Could you check a few things on this model? Use its own coordinates, in mm. A direction names the side the tool comes from. Give positions to 0.01 mm unless a question says otherwise; leave off trailing zeros. Loops run counter-clockwise (first coordinate to the right, second up) from the corner with the lowest first, then second, coordinate; pieces in that order, holes last. Notation, with made-up numbers: (38.5, 39.25) -> (77.5, 39.25) arc R9 ccw to (77.5, 54.25) -> close; hole circle Ø4 at (39, -16.75). An arc over 180 degrees is marked (long way). Put each result on its own line as item: value.
```python
from build123d import *

# Parameters (mm, degrees)
SKETCH_1_W               = 90
SKETCH_1_H               = 65
EXTRUDE_1_DEPTH          = 2
SKETCH_2_W               = 52
SKETCH_2_H               = 13
CUT_EXTRUDE_1_DEPTH      = 56.54502678
CUT_EXTRUDE_2_DEPTH      = 56.54502678
MIRROR_3_COPY_1_DEPTH    = 56.54502678
FILLET_1_R               = 7
SKETCH_4_W               = 41
SKETCH_4_H               = 2
EXTRUDE_2_DEPTH          = 73
SKETCH_5_W               = 15
SKETCH_5_H               = 59.991373208
CUT_EXTRUDE_3_DEPTH      = 0.5
FILLET_2_R               = 0.5
FILLET_3_R               = 0.5
CHAMFER_4_SIZE           = 12
CHAMFER_4_SIZE2          = 25.734083046
CHAMFER_5_SIZE           = 12
CHAMFER_5_SIZE2          = 25.734083046
CHAMFER_6_SIZE           = 12
CHAMFER_6_SIZE2          = 25.734083046
CHAMFER_7_SIZE           = 12
CHAMFER_7_SIZE2          = 25.734083046
FILLET_4_R               = 10
EXTRUDE_3_DEPTH          = 6
EXTRUDE_START            = -41
SKETCH_7_R               = 4
EXTRUDE_4_DEPTH          = 42
SKETCH_8_R               = 2.75
CUT_EXTRUDE_4_DEPTH      = 92.707415265
MIRROR_9_COPY_1_SKETCH_R = 2.75
MIRROR_9_COPY_1_DEPTH    = 92.707415265
EXTRUDE_7_DEPTH          = 13
EXTRUDE_7_DEPTH_BACK     = 13
SKETCH_10_R              = 37.5
FILLET_5_R               = 2
SKETCH_11_R              = 25
SKETCH_11_R_2            = 22
CUT_EXTRUDE_5_DEPTH      = 3
FILLET_6_R               = 2
FILLET_7_R               = 2
CHAMFER_8_SIZE2          = 5.196152423
CHAMFER_8_SIZE           = 3
CHAMFER_9_SIZE2          = 3
CHAMFER_9_SIZE           = 5.196152423


with BuildPart() as part:
    # 草图1 → 凸台-拉伸1 (new body)
    with BuildSketch(Plane.XY):
        Rectangle(SKETCH_1_W, SKETCH_1_H)
    extrude(amount=EXTRUDE_1_DEPTH)

    # 草图2 → 切除-拉伸1 (cut, through all)
    with BuildSketch(Plane.XY.offset(2)):
        with Locations((0, 26)):
            Rectangle(SKETCH_2_W, SKETCH_2_H)
    cut_extrude_1 = extrude(amount=-CUT_EXTRUDE_1_DEPTH, mode=Mode.SUBTRACT)

    # 镜向1: 切除-拉伸1 across plane
    add(cut_extrude_1.mirror(Plane.ZX), mode=Mode.SUBTRACT)

    # 草图3 → 切除-拉伸2 (cut, through all)
    with BuildSketch(Plane.XY.offset(2)):
        with BuildLine():
            Line((-36.562223186, 30.159744382), (-34.562223186, 30.159744382))
            ThreePointArc((-34.562223186, 30.159744382), (-30.562223186, 26.159744382), (-34.562223186, 22.159744382))
            Line((-34.562223186, 22.159744382), (-36.562223186, 22.159744382))
            ThreePointArc((-36.562223186, 22.159744382), (-40.562223186, 26.159744382), (-36.562223186, 30.159744382))
        make_face()
    cut_extrude_2 = extrude(amount=-CUT_EXTRUDE_2_DEPTH, mode=Mode.SUBTRACT)

    # 镜向2: 切除-拉伸2 across plane
    add(cut_extrude_2.mirror(Plane(origin=(0, 0, 0), x_dir=(0, 0, 1), z_dir=(1, 0, 0))), mode=Mode.SUBTRACT)

    # 镜向3: 切除-拉伸2 across plane
    add(cut_extrude_2.mirror(Plane.ZX), mode=Mode.SUBTRACT)

    # 镜向3 copy 1 sketch → 镜向3 copy 1 (cut, through all)
    with BuildSketch(Plane(origin=(0, 0, 2), x_dir=(-1, 0, 0), z_dir=(0, 0, 1))):
        with BuildLine():
            Line((-36.562223186, 30.159744382), (-34.562223186, 30.159744382))
            ThreePointArc((-34.562223186, 30.159744382), (-30.562223186, 26.159744382), (-34.562223186, 22.159744382))
            Line((-34.562223186, 22.159744382), (-36.562223186, 22.159744382))
            ThreePointArc((-36.562223186, 22.159744382), (-40.562223186, 26.159744382), (-36.562223186, 30.159744382))
        make_face()
    extrude(amount=-MIRROR_3_COPY_1_DEPTH, mode=Mode.SUBTRACT)

    # 圆角1
    fillet_1_edges = [part.edges().sort_by_distance(p)[0] for p in [
        (-26, 32.5, 1),
        (26, 32.5, 1),
        (-26, -32.5, 1),
        (26, -32.5, 1),
        (45, -32.5, 1),
        (-45, -32.5, 1),
        (-45, 32.5, 1),
        (45, 32.5, 1),
    ]]
    fillet(fillet_1_edges, radius=FILLET_1_R)

    # 草图4 → 凸台-拉伸2 (add)
    with BuildSketch(Plane(origin=(0, 0, 0), x_dir=(-1, 0, 0), z_dir=(0, 0, -1))):
        with Locations((0, 18.5)):
            Rectangle(SKETCH_4_W, SKETCH_4_H)
    extrude_2 = extrude(amount=EXTRUDE_2_DEPTH)

    # 镜向4: 凸台-拉伸2 across plane
    add(extrude_2.mirror(Plane.ZX))

    # 草图5 → 切除-拉伸3 (cut)
    with BuildSketch(Plane(origin=(0, 19.5, 0), x_dir=(1, 0, 0), z_dir=(0, 1, 0))):
        with Locations((0, 43.004313396)):
            Rectangle(SKETCH_5_W, SKETCH_5_H)
    cut_extrude_3 = extrude(amount=-CUT_EXTRUDE_3_DEPTH, mode=Mode.SUBTRACT)

    # 圆角2
    fillet_2_edges = [part.edges().sort_by_distance(p)[0] for p in [
        (0, 19.5, -13.008626792),
        (7.5, 19.5, -43.004313396),
        (-7.5, 19.5, -43.004313396),
    ]]
    fillet(fillet_2_edges, radius=FILLET_2_R - 0.0001)  # a hair under: the kernel refuses the full size

    # 镜向6: 切除-拉伸3 across plane
    add(cut_extrude_3.mirror(Plane.ZX), mode=Mode.SUBTRACT)

    # 圆角3
    fillet_3_edges = [part.edges().sort_by_distance(p)[0] for p in [
        (7.5, -19.5, -43.004313396),
        (-7.5, -19.5, -43.004313396),
        (0, -19.5, -13.008626792),
    ]]
    fillet(fillet_3_edges, radius=FILLET_3_R - 0.0001)  # a hair under: the kernel refuses the full size

    # 倒角4
    chamfer_4_edges = [part.edges().sort_by_distance(p)[0] for p in [
        (-20.5, -18.5, -73),
    ]]
    chamfer_4_side = [part.faces().sort_by_distance(p)[0] for p in [
        (0, -18.423106996, -73),
    ]]
    chamfer(chamfer_4_edges, length=CHAMFER_4_SIZE, length2=CHAMFER_4_SIZE2, reference=chamfer_4_side[0])

    # 倒角5
    chamfer_5_edges = [part.edges().sort_by_distance(p)[0] for p in [
        (20.5, -18.5, -73),
    ]]
    chamfer_5_side = [part.faces().sort_by_distance(p)[0] for p in [
        (6.905756389, -18.386486006, -73),
    ]]
    chamfer(chamfer_5_edges, length=CHAMFER_5_SIZE, length2=CHAMFER_5_SIZE2, reference=chamfer_5_side[0])

    # 倒角6
    chamfer_6_edges = [part.edges().sort_by_distance(p)[0] for p in [
        (20.5, 18.5, -73),
    ]]
    chamfer_6_side = [part.faces().sort_by_distance(p)[0] for p in [
        (0, 18.423106996, -73),
    ]]
    chamfer(chamfer_6_edges, length=CHAMFER_6_SIZE, length2=CHAMFER_6_SIZE2, reference=chamfer_6_side[0])

    # 倒角7
    chamfer_7_edges = [part.edges().sort_by_distance(p)[0] for p in [
        (-20.5, 18.5, -73),
    ]]
    chamfer_7_side = [part.faces().sort_by_distance(p)[0] for p in [
        (-6.905756389, 18.386486006, -73),
    ]]
    chamfer(chamfer_7_edges, length=CHAMFER_7_SIZE, length2=CHAMFER_7_SIZE2, reference=chamfer_7_side[0])

    # 圆角4
    fillet_4_edges = [part.edges().sort_by_distance(p)[0] for p in [
        (-8.5, 18.5, -73),
        (8.5, 18.5, -73),
        (8.5, -18.5, -73),
        (-8.5, -18.5, -73),
    ]]
    fillet(fillet_4_edges, radius=FILLET_4_R)

    # 草图6 → 凸台-拉伸3 (add)
    with BuildSketch(Plane(origin=(0, 19, 0), x_dir=(1, 0, 0), z_dir=(0, 1, 0))):
        Polygon((-4.39108988, 69.342635878), (-7.986809677, 62.196252237), (-3.595719796, 55.509075728), (4.39108988, 55.96828286), (7.986809677, 63.114666501), (3.595719796, 69.801843011), align=None)
    extrude_3 = extrude(amount=EXTRUDE_3_DEPTH)

    # 草图7 → 凸台-拉伸4 (add)
    with BuildSketch(Plane(origin=(0, 25, 0), x_dir=(1, 0, 0), z_dir=(0, 1, 0)).offset(EXTRUDE_START)):
        with Locations(Location((0, 62.655459369, 0), (0, 0, 270))):
            Circle(SKETCH_7_R)
    extrude_4 = extrude(amount=EXTRUDE_4_DEPTH)

    # 镜向7: 凸台-拉伸3, 凸台-拉伸4 across plane
    add(extrude_3.mirror(Plane.ZX))
    add(extrude_4.mirror(Plane.ZX))

    # 草图8 → 切除-拉伸4 (cut, through all)
    with BuildSketch(Plane(origin=(0, 0, 0), x_dir=(-1, 0, 0), z_dir=(0, 0, -1))):
        with Locations((-23.25, 19.5)):
            Circle(SKETCH_8_R)
    cut_extrude_4 = extrude(amount=-CUT_EXTRUDE_4_DEPTH, mode=Mode.SUBTRACT)

    # 镜向8: 切除-拉伸4 across plane
    add(cut_extrude_4.mirror(Plane.ZX), mode=Mode.SUBTRACT)

    # 镜向9: 切除-拉伸4 across plane
    add(cut_extrude_4.mirror(Plane(origin=(0, 0, 0), x_dir=(0, 0, 1), z_dir=(1, 0, 0))), mode=Mode.SUBTRACT)

    # 镜向9 copy 1 sketch → 镜向9 copy 1 (cut, through all)
    with BuildSketch(Plane(origin=(0, 0, 0), x_dir=(1, 0, 0), z_dir=(0, 0, -1))):
        with Locations((-23.25, 19.5)):
            Circle(MIRROR_9_COPY_1_SKETCH_R)
    extrude(amount=-MIRROR_9_COPY_1_DEPTH, mode=Mode.SUBTRACT)

    # 草图10 → 凸台-拉伸7 (add, two sides: drawn at the far end of the back side and taken through both)
    with BuildSketch(Plane(origin=(0, 0, 0), x_dir=(1, 0, 0), z_dir=(0, 1, 0)).offset(-EXTRUDE_7_DEPTH_BACK)):
        with Locations(Location((0, 62.655459369, 0), (0, 0, 270))):
            Circle(SKETCH_10_R)
    extrude(amount=EXTRUDE_7_DEPTH + EXTRUDE_7_DEPTH_BACK)

    # 圆角5
    fillet_5_edges = [part.edges().sort_by_distance(p)[0] for p in [
        (0, -13, -100.155459369),
        (0, 13, -100.155459369),
    ]]
    fillet(fillet_5_edges, radius=FILLET_5_R)

    # 草图11 → 切除-拉伸5 (cut)
    with BuildSketch(Plane(origin=(0, 13, 0), x_dir=(1, 0, 0), z_dir=(0, 1, 0))):
        with Locations(Location((0, 62.655459369, 0), (0, 0, 270))):
            Circle(SKETCH_11_R)
        with Locations(Location((0, 62.655459369, 0), (0, 0, 270))):
            Circle(SKETCH_11_R_2, mode=Mode.SUBTRACT)
    cut_extrude_5 = extrude(amount=-CUT_EXTRUDE_5_DEPTH, mode=Mode.SUBTRACT)

    # 圆角6
    fillet_6_edges = [part.edges().sort_by_distance(p)[0] for p in [
        (0, 13, -87.655459369),
    ]]
    fillet(fillet_6_edges, radius=FILLET_6_R)

    # 镜向10: 切除-拉伸5 across plane
    add(cut_extrude_5.mirror(Plane.ZX), mode=Mode.SUBTRACT)

    # 圆角7
    fillet_7_edges = [part.edges().sort_by_distance(p)[0] for p in [
        (0, -13, -87.655459369),
    ]]
    fillet(fillet_7_edges, radius=FILLET_7_R)

    # 倒角8
    chamfer_8_edges = [part.edges().sort_by_distance(p)[0] for p in [
        (0, 13, -84.655459369),
    ]]
    chamfer_8_side = [part.faces().sort_by_distance(p)[0] for p in [
        (0, 12.94, -84.655459369),
    ]]
    chamfer(chamfer_8_edges, length=CHAMFER_8_SIZE - 0.0001, length2=CHAMFER_8_SIZE2 - 0.0001, reference=chamfer_8_side[0])  # a hair under: the kernel refuses the full size

    # 倒角9
    chamfer_9_edges = [part.edges().sort_by_distance(p)[0] for p in [
        (0, -13, -84.655459369),
    ]]
    chamfer_9_side = [part.faces().sort_by_distance(p)[0] for p in [
        (0, -13, -84.595459369),
    ]]
    chamfer(chamfer_9_edges, length=CHAMFER_9_SIZE - 0.0001, length2=CHAMFER_9_SIZE2 - 0.0001, reference=chamfer_9_side[0])  # a hair under: the kernel refuses the full size


solid = part.part
```
1. If we section it at B-B (z = -54): Count the separate pieces of the cut face and the enclosed holes in it, then the cut area to 3 significant figures.
Recorded:
separate pieces: 3
enclosed holes: 0
area: 1,940 mm^2
2. I need wall thicknesses on line 1 (Y direction, x = -19.5, z = -35.5); line 2 (Y direction, x = -13, z = -5); line 3 (Y direction, x = 4.5, z = -69.5). Which ranges of each line are inside material? Lowest first, please.
Recorded:
line 1: y = -19.5 to -17.5, -13 to 13, 17.5 to 19.5
line 2: y = -19.5 to -17.5, 17.5 to 19.5
line 3: y = -19 to -17.5, -13 to 13, 17.5 to 19
3. For faces 4 (the face through (-28.1, -30.5, 1)), 5 (the face through (0.18, 15.22, -66.65)), 6 (the face through (-4, 25, -64)), 7 (the face through (0, -19, -70)), which set-ups out of +Z, -Z, +X, -X, +Y, -Y let a thin tool reach every point of the face, with its end or its side?
Recorded:
face 4: +Z, -Z, -Y
face 5: none
face 6: +Y
face 7: -Z, -Y
4. Thinking about a two-plate mould opening in X: for faces 1 (the face through (-3, -13, -59)), 2 (the face through (-10.378, 12.854, -76.191)), 3 (the face through (42.9, 30.5, 1)), which applies, pulls with the +X half, pulls with the -X half, needs draft (parallel to the pull), parting line crosses it, or undercut?
Recorded:
face 1: needs draft
face 2: undercut
face 3: pulls with the +X half
5. If we section it at A-A (y = 2.5): List the corners of the cut face in (x, z) for me, then the cut area to 3 significant figures.
Recorded:
outline: (-45, 0) -> (45, 0) -> (45, 2) -> (-45, 2) -> close; circle Ø75 at (0, -62.66)
area: 4,600 mm^2
6. I'm going to push flat-ended pins straight in: pin 1 (8 mm diameter, centred on x = 36, z = -54.5, fed in from +Y); pin 2 (3 mm diameter, centred on x = -13.5, z = -23.5, fed in from -Y); pin 3 (11 mm diameter, centred on x = -2, z = -68.5, fed in from -Y). Where does each tip first touch, or does it pass through?
Recorded:
pin 1: stops at y = 13
pin 2: stops at y = -19.5
pin 3: stops at y = -26
